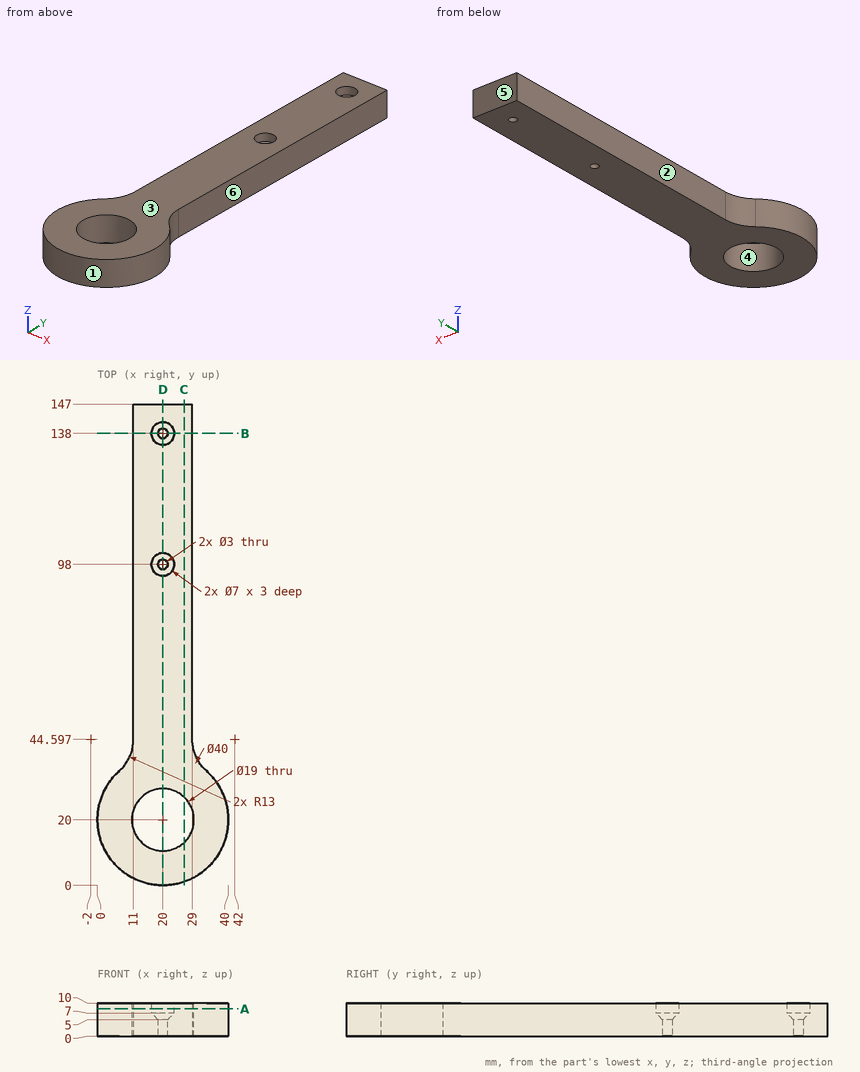
Here's the drawing with two shaded views (mm, measured from the low corner). I have some questions. A direction names the side the tool comes from. Coordinates: 2 decimals unless noted, no trailing zeros. Loops run counter-clockwise (first coordinate to the right, second up) from the corner with the lowest first, then second, coordinate; pieces in that order, holes last. Notation, with made-up numbers: (70.25, 37.5) -> (95.25, 37.5) arc R21 cw to (95.25, 70.5) -> close; hole circle Ø3 at (89.5, 16.25). An arc over 180 degrees is marked (long way). Put each result on its own line as item: value. Start each with the question number.
Q1. I want a section at D-D (x = 20). Write out the boundary of the cut face in (y, z).
Q2. Thinking about a two-plate mould opening in X: for the marked faces 1, 2, 3 and 4, which applies, pulls with the +X half, pulls with the -X half, needs draft (parallel to the pull), parting line crosses it, or undercut?
Q3. I want a section at B-B (y = 138). Write out the boundary of the cut face in (x, z), plus the area to 3 significant figures.
Q4. I want a section at A-A (z = 8.25). Write out the boundary of the cut face in (x, y).
Q5. I'm going to push flat-ended pins straight in: P1, Ø3, axis at y = 131.5, z = 5, coming from the +X side; P2, Ø5, axis at y = 117.5, z = 3, coming from the -X side; P3, Ø2.5, axis at x = 20, y = 98, coming from the -Z side; P4, Ø2, axis at x = 25.5, z = 5.5, coming from the -Y side. Where does each tip first touch, or does it pass through?
Q6. For the marked faces 5 and 6, which set-ups out of +Z, -Z, +X, -X, +Y, -Y let a thin tool reach every point of the face, with its end or its side?
Q7. If I drill on line 1 (Y direction, x = 20, z = 8.1); line 2 (Y direction, x = 20, z = 6.25); line 3 (X direction, y = 98, z = 3.05), over which ranges is the centre line in solid material (lowest first)? Write a range as [from, to].
Q8. I want a section at C-C (x = 26.5). Write out the boundary of the cut face in (y, z).
Taken from the geometry:
1. outline: (0, 0) -> (10.5, 0) -> (10.5, 10) -> (0, 10) -> close; (29.5, 0) -> (96.5, 0) -> (96.5, 5) -> (94.5, 7) -> (94.5, 10) -> (29.5, 10) -> close; (99.5, 0) -> (136.5, 0) -> (136.5, 5) -> (134.5, 7) -> (134.5, 10) -> (101.5, 10) -> (101.5, 7) -> (99.5, 5) -> close; (139.5, 0) -> (147, 0) -> (147, 10) -> (141.5, 10) -> (141.5, 7) -> (139.5, 5) -> close
2. face 1: parting line crosses it
2. face 2: pulls with the -X half
2. face 3: needs draft
2. face 4: undercut
3. outline: (11, 0) -> (18.5, 0) -> (18.5, 5) -> (16.5, 7) -> (16.5, 10) -> (11, 10) -> close; (21.5, 0) -> (29, 0) -> (29, 10) -> (23.5, 10) -> (23.5, 7) -> (21.5, 5) -> close
3. area: 134 mm2
4. outline: (6.67, 34.91) arc R20 ccw (long way) to (33.33, 34.91) arc R13 cw to (29, 44.6) -> (29, 147) -> (11, 147) -> (11, 44.6) arc R13 cw to start; hole circle Ø19 at (20, 20); hole circle Ø7 at (20, 98); hole circle Ø7 at (20, 138)
5. P1: stops at x = 29
5. P2: stops at x = 11
5. P3: passes through
5. P4: stops at y = 0.51
6. face 5: +Z, -Z, +X, -X, +Y
6. face 6: +Z, -Z, +X, +Y
7. line 1: y = [0, 10.5], [29.5, 94.5], [101.5, 134.5], [141.5, 147]
7. line 2: y = [0, 10.5], [29.5, 95.25], [100.75, 135.25], [140.75, 147]
7. line 3: x = [11, 18.5], [21.5, 29]
8. outline: (1.09, 0) -> (13.07, 0) -> (13.07, 10) -> (1.09, 10) -> close; (26.93, 0) -> (147, 0) -> (147, 10) -> (26.93, 10) -> close
